```python
from build123d import *
from OCP.BRepAlgoAPI import BRepAlgoAPI_Cut
from OCP.TopTools import TopTools_ListOfShape

# Parameters (mm, degrees)
SKETCH1_W               = 22.054431489
SKETCH1_H               = 12.5
BOSS_EXTRUDE1_DEPTH     = 40
CUT_EXTRUDE1_DEPTH      = 10
CUT_EXTRUDE1_DEPTH_BACK = 15
SKETCH2_R               = 1.5
FILLET3_START           = -1
FILLET3_DEPTH           = 36.616951747
FILLET3_START_2         = -31
FILLET3_2_DEPTH         = 14
SKETCH5_R               = 1.5
CUT_EXTRUDE4_DEPTH      = 53.866443736
SKETCH16_W              = 22.05443149
SKETCH16_H              = 2
CUT_EXTRUDE6_DEPTH      = 8.5
FILLET4_R               = 2


with BuildPart() as part:
    # Sketch1 → Boss-Extrude1 (new body)
    with BuildSketch(Plane.XY):
        with Locations((-13.228930986, -24.070183414)):
            Rectangle(SKETCH1_W, SKETCH1_H)
    extrude(amount=BOSS_EXTRUDE1_DEPTH)

    # Sketch2 → Cut-Extrude1 (cut, two sides: drawn at the far end of the back side and taken through both)
    with BuildSketch(Plane.XZ.offset(30.320183414).offset(-CUT_EXTRUDE1_DEPTH_BACK)):
        with Locations(Location((-13.228930986, 6.5, 0), (0, 0, 90))):
            Circle(SKETCH2_R)
        with Locations(Location((-13.228930986, 31.5, 0), (0, 0, 90))):
            Circle(SKETCH2_R)
        with BuildLine():
            Line((-4.478930986, 29.25), (-2.201715242, 29.25))
            add(Edge.make_bspline(
                [(-24.256146731, 29.25), (-34.277912729, 38.417119108), (-13.227499763, 50.308047167), (7.840407292, 38.416977249), (-2.201715242, 29.25)],
                knots=[0, 0, 0, 0, 0.49986218, 1, 1, 1, 1], degree=3))
            add(Edge.make_bspline(
                [(-6.103895584, 34.329012749), (-10.720559386, 33.527203043), (-28.641384523, 40.845191705), (-24.256146731, 29.25)],
                knots=[0, 0, 0, 0, 1, 1, 1, 1], degree=3))
            ThreePointArc((-6.103895584, 34.329012749), (-4.895067543, 31.916312081), (-4.478930986, 29.25))
        make_face()
        with BuildLine():
            Line((-4.478930986, 8.75), (-2.201715242, 8.75))
            add(Edge.make_bspline(
                [(-2.201715242, 8.75), (5.39210746, 3.880294823), (-0.777052631, -4.523329032), (-17.174300591, -10.623347238), (-34.821400648, -0.026005424), (-24.256146731, 8.75)],
                knots=[0, 0, 0, 0, 0.283272691, 0.504244858, 1, 1, 1, 1], degree=3))
            add(Edge.make_bspline(
                [(-23.490579314, 0), (-24.966512963, 4.237786421), (-24.256146731, 8.75)],
                knots=[0, 0, 0, 1, 1, 1], degree=2))
            Line((-23.490579314, 0), (-13.228930986, 0))
            ThreePointArc((-13.228930986, 0), (-7.041746651, 2.562815665), (-4.478930986, 8.75))
        make_face()
    extrude(amount=CUT_EXTRUDE1_DEPTH + CUT_EXTRUDE1_DEPTH_BACK, mode=Mode.SUBTRACT)


with BuildPart() as fillet3_tool:
    # Fillet3: read off the stored shape, not the designer's step
    # Fillet3 outline → Fillet3 (new body)
    with BuildSketch(Plane.XY.offset(FILLET3_START)):
        with BuildLine():
            Line((-24.256146731, -17.820183414), (-24.256146731, -19.820183414))
            ThreePointArc((-24.256146731, -19.820183414), (-23.670360293, -18.405969851), (-22.256146731, -17.820183414))
            Line((-22.256146731, -17.820183414), (-24.256146731, -17.820183414))
        make_face()
        with BuildLine():
            ThreePointArc((-22.256146731, -30.320183414), (-23.670360293, -29.734396976), (-24.256146731, -28.320183414))
            Line((-24.256146731, -28.320183414), (-24.256146731, -30.320183414))
            Line((-24.256146731, -30.320183414), (-22.256146731, -30.320183414))
        make_face()
    extrude(amount=FILLET3_DEPTH)


with BuildPart() as part_1:
    add(part.part)

    # Fillet3: cut by fillet3_tool, with a tolerance
    fillet3_stock = TopTools_ListOfShape()
    fillet3_stock.Append(part_1.part.wrapped)
    fillet3_tools = TopTools_ListOfShape()
    fillet3_tools.Append(fillet3_tool.part.wrapped)
    fillet3_cut = BRepAlgoAPI_Cut()
    fillet3_cut.SetArguments(fillet3_stock)
    fillet3_cut.SetTools(fillet3_tools)
    fillet3_cut.SetFuzzyValue(0.00001)
    fillet3_cut.Build()
    add(Compound.cast(fillet3_cut.Shape()).solids(), mode=Mode.REPLACE)


with BuildPart() as fillet3_2_tool:
    # Fillet3 2 outline → Fillet3 2 (new body)
    with BuildSketch(Plane(origin=(0, 0, 0), x_dir=(1, 0, 0), z_dir=(0, 1, 0)).offset(FILLET3_START_2)):
        with BuildLine():
            Line((-24.256146731, -3.001504812), (-24.256146731, -3.16929397))
            ThreePointArc((-24.256146731, -3.16929397), (-24.248700679, -2.996873655), (-24.226417966, -2.82573719))
            add(Edge.make_bspline(
                [(-24.226417966, -2.82573719), (-24.241732441, -2.913564505), (-24.256146731, -3.001504812)],
                knots=[0.329874436, 0.329874436, 0.329874436, 0.350165787, 0.350165787, 0.350165787], degree=2))
        make_face()
        with BuildLine():
            ThreePointArc((-23.055175533, -35.347858737), (-23.929176558, -34.610293214), (-24.256146731, -33.5144049))
            Line((-24.256146731, -33.5144049), (-24.256146731, -34.486377393))
            add(Edge.make_bspline(
                [(-24.256146731, -34.486377393), (-23.945543724, -34.85491353), (-23.538709887, -35.137131928), (-23.055175533, -35.347858737)],
                knots=[0.223074816, 0.223074816, 0.223074816, 0.223074816, 0.304929745, 0.304929745, 0.304929745, 0.304929745], degree=3))
        make_face()
    extrude(amount=FILLET3_2_DEPTH)


with BuildPart() as part_2:
    add(part_1.part)

    # Fillet3 2: cut by fillet3_2_tool, with a tolerance
    fillet3_2_stock = TopTools_ListOfShape()
    fillet3_2_stock.Append(part_2.part.wrapped)
    fillet3_2_tools = TopTools_ListOfShape()
    fillet3_2_tools.Append(fillet3_2_tool.part.wrapped)
    fillet3_2_cut = BRepAlgoAPI_Cut()
    fillet3_2_cut.SetArguments(fillet3_2_stock)
    fillet3_2_cut.SetTools(fillet3_2_tools)
    fillet3_2_cut.SetFuzzyValue(0.00001)
    fillet3_2_cut.Build()
    add(Compound.cast(fillet3_2_cut.Shape()).solids(), mode=Mode.REPLACE)

    # Sketch5 → Cut-Extrude4 (cut, through all)
    with BuildSketch(Plane.XY):
        with Locations(Location((-18.011106811, -24.070183414, 0), (0, 0, 180))):
            Circle(SKETCH5_R)
        with Locations(Location((-8.446755162, -24.070183414, 0), (0, 0, 180))):
            Circle(SKETCH5_R)
    extrude(amount=CUT_EXTRUDE4_DEPTH, mode=Mode.SUBTRACT)

    # Sketch16 → Cut-Extrude6 (cut)
    with BuildSketch(Plane.XY.offset(38)):
        with Locations((-13.228930985, -20.1809771)):
            Rectangle(SKETCH16_W, SKETCH16_H)
        with Locations((-13.228930985, -28.261916897)):
            Rectangle(SKETCH16_W, SKETCH16_H)
    extrude(amount=-CUT_EXTRUDE6_DEPTH, mode=Mode.SUBTRACT)

    # Fillet4
    # the kernel refuses this fillet: 2 mm, written as the material it takes off along each edge
    with BuildSketch(Plane(origin=(-6.103895584, -22.583679851, 34.329012749), x_dir=(0.5153680546007453, 0, -0.8569689424343471), z_dir=(0, 1, 0))) as fillet4_piece_1:
        with BuildLine():
            CenterArc((1.205528974, 1.993941708), FILLET4_R, 212.228268917, 62.232476225)
            Line((-0.486331325, 0.927354287), (-0.520168531, 0.906022538))
            ThreePointArc((-0.520168531, 0.906022538), (-0.25689069, 0.456334761), (-0.037300681, -0.01444504))
            Line((-0.037300681, -0.01444504), (-0.003111043, -0.039878834))
            ThreePointArc((-0.003111043, -0.039878834), (0.68054055, -0.066505026), (1.364192143, -0.039878834))
            Line((1.364192143, -0.039878834), (1.3610811, 0))
        make_face()
    extrude(amount=8.166199187, mode=Mode.SUBTRACT)
    with BuildSketch(Plane(origin=(-6.103895584, -30.664619647, 34.329012749), x_dir=(0.5153680546007453, 0, -0.8569689424343471), z_dir=(0, 1, 0))) as fillet4_piece_2:
        with BuildLine():
            CenterArc((1.205528974, 1.993941708), FILLET4_R, 212.228268917, 62.232476225)
            Line((-0.486331325, 0.927354287), (-0.520168531, 0.906022538))
            ThreePointArc((-0.520168531, 0.906022538), (-0.25689069, 0.456334761), (-0.037300681, -0.01444504))
            Line((-0.037300681, -0.01444504), (-0.003111043, -0.039878834))
            ThreePointArc((-0.003111043, -0.039878834), (0.68054055, -0.066505026), (1.364192143, -0.039878834))
            Line((1.364192143, -0.039878834), (1.3610811, 0))
        make_face()
    extrude(amount=12.886345297, mode=Mode.SUBTRACT)
    with BuildSketch(Plane(origin=(-6.103895584, -33.722886164, 34.329012749), x_dir=(0.5153680546007453, 0, -0.8569689424343471), z_dir=(0, 1, 0))) as fillet4_piece_3:
        with BuildLine():
            CenterArc((1.205528974, 1.993941708), FILLET4_R, 212.228268917, 62.232476225)
            Line((-0.486331325, 0.927354287), (-0.520168531, 0.906022538))
            ThreePointArc((-0.520168531, 0.906022538), (-0.25689069, 0.456334761), (-0.037300681, -0.01444504))
            Line((-0.037300681, -0.01444504), (-0.003111043, -0.039878834))
            ThreePointArc((-0.003111043, -0.039878834), (0.68054055, -0.066505026), (1.364192143, -0.039878834))
            Line((1.364192143, -0.039878834), (1.3610811, 0))
        make_face()
    extrude(amount=7.863672018, mode=Mode.SUBTRACT)


solid = part_2.part
```
Can you work these out from the model? Positions are in its coordinate system, mm. A direction names the side the tool comes from. Coordinates: 2 decimals unless noted, no trailing zeros. Order: outer loops, then holes, each group sorted by start corner. A loop starts at its lowest first (then second) coordinate and runs counter-clockwise, first axis right, second up. Notation, with made-up numbers: (32.5, -8) - (70.5, -8) arc R20 ccw to (70.5, 6) - close; hole circle Ø1 at (-19.5, -15). An arc over 180 degrees is marked (long way). Answer in a Markdown table with one row per item.
1. For faces 4 (the flat face through (-3, -24, 8.75)), 5 (the flat face through (-3, -24, 29.25)), 6 (the flat face through (-15, -28, 29.5)), 7 (the flat face through (-20, -24, 0)), 8 (the flat face through (-12, -30.32, 18)), which set-ups out of +Z, -Z, +X, -X, +Y, -Y let a thin tool reach every point of the face, with its end or its side?
Reply:
| item | result |
|---|---|
| face 4 | -Z, +X, +Y, -Y |
| face 5 | +Z, +X, +Y, -Y |
| face 6 | +Z, +X, -X |
| face 7 | -Z, +X, -X, +Y, -Y |
| face 8 | +Z, -Z, +X, -X, -Y |
2. If I drill on line 1 along Y through (x, z) = (-14.75, 32); line 2 along X through (y, z) = (-24.75, 20.5); line 3 along Z through (x, y) = (-13, -25.75), over which ranges is the centre line in solid material (lowest first)?
Reply:
| item | result |
|---|---|
| line 1 | y = -30.32 to -29.26, -27.26 to -21.18, -19.18 to -17.82 |
| line 2 | x = -24.26 to -19.35, -16.67 to -9.78, -7.11 to -2.2 |
| line 3 | z = 0 to 5.02, 7.98 to 30.02, 32.98 to 35.09 |
3. Suppose I cut it at D-D (z = 13.5). Please give me the cut outline in (x, y).
Reply:
| item | result |
|---|---|
| outline | (-24.26, -28.32) arc R2 ccw to (-22.26, -30.32) - (-2.2, -30.32) - (-2.2, -17.82) - (-22.26, -17.82) arc R2 ccw to (-24.26, -19.82) - close; hole circle Ø3 at (-18.01, -24.07); hole circle Ø3 at (-8.45, -24.07) |
4. Suppose I cut it at A-A (z = 31.5). Please give me the cut outline in (x, y), and give its area (3 significant figures).
Reply:
| item | result |
|---|---|
| outline | (-24.26, -27.26) - (-14.73, -27.26) - (-14.73, -21.18) - (-24.26, -21.18) - close; (-24.15, -19.18) - (-14.73, -19.18) - (-14.73, -17.82) - (-22.26, -17.82) arc R2 ccw to start; (-24.02, -29.26) arc R2 ccw to (-22.26, -30.32) - (-14.73, -30.32) - (-14.73, -29.26) - close; (-11.73, -30.32) - (-4.77, -30.32) - (-4.77, -29.26) - (-11.73, -29.26) - close; (-11.73, -27.26) - (-4.77, -27.26) - (-4.77, -21.18) - (-11.73, -21.18) - close; (-11.73, -19.18) - (-4.77, -19.18) - (-4.77, -17.82) - (-11.73, -17.82) - close; hole circle Ø3 at (-18.01, -24.07); hole circle Ø3 at (-8.45, -24.07) |
| area | 124 mm^2 |
5. Suppose I cut it at C-C (x = -3.75). Please give me the cut outline in (y, z), and give its area (3 significant figures).
Reply:
| item | result |
|---|---|
| outline | (-30.32, 8.75) - (-17.82, 8.75) - (-17.82, 29.25) - (-30.32, 29.25) - close |
| area | 256 mm^2 |
6. For pin 1 (3.5 mm diameter, centred on x = -8.45, y = -24.07, fed in from +Z); pin 2 (2 mm diameter, centred on x = -12, y = -28, fed in from +Z); pin 3 (2 mm diameter, centred on x = -11, y = -20, fed in from +Z), each with a flat end and sliding along its axis, tell me the tip position at first contact or that it passes through.
Reply:
| item | result |
|---|---|
| pin 1 | stops at z = 34.61 |
| pin 2 | stops at z = 35.03 |
| pin 3 | stops at z = 34.84 |
7. Suppose I cut it at B-B (z = 6.5). Please give me the cut outline in (x, y).
Reply:
| item | result |
|---|---|
| outline | (-24.26, -28.32) arc R2 ccw to (-22.26, -30.32) - (-14.73, -30.32) - (-14.73, -17.82) - (-22.26, -17.82) arc R2 ccw to (-24.26, -19.82) - close; (-11.73, -30.32) - (-4.77, -30.32) - (-4.77, -17.82) - (-11.73, -17.82) - close; hole circle Ø3 at (-18.01, -24.07); hole circle Ø3 at (-8.45, -24.07) |
8. If we mould it in two halves opening along X, with no side actions, what happens to faces 1 (the cylindrical face through (-23.92, -24.264, 34.624)), 2 (the flat face through (-2.202, -24, 19)), 3 (the cylindrical face through (-13.3, -18.5, 30))? For each: pulls with the +X half, pulls with the -X half, needs draft (parallel to the pull), parting line crosses it, or undercut.
Reply:
| item | result |
|---|---|
| face 1 | pulls with the -X half |
| face 2 | pulls with the +X half |
| face 3 | undercut |
